Geometry check sheet. Reference: drawing and pictorial views, mm from the part's lowest x, y, z. A direction names the side the tool comes from. Give positions to 0.01 mm unless a question says otherwise; leave off trailing zeros. Loops run counter-clockwise (first coordinate to the right, second up) from the corner with the lowest first, then second, coordinate; pieces in that order, holes last. Notation, with made-up numbers: (-30, 1.5) - (-3, 1.5) arc R15 cw to (-3, 9.5) - close; hole circle Ø6 at (17.25, 16). An arc over 180 degrees is marked (long way). Answer in a Markdown table with one row per item. Add a question column.
(1) Sectioned sample at D-D on x = 28. Enter the section's corners in (y, z).
(2) Set-up check for the marked faces 1 and 2: record each of +Z, -Z, +X, -X, +Y, -Y from which the full face is reachable in a straight line by a thin tool's end or side.
(3) Draft check along Z on the marked faces 3, 4 and 5. Enter one of: released by +Z, released by -Z, zero draft, split by the parting line, or undercut.
(4) Sectioned sample at B-B on x = 16. Enter the section's corners in (y, z).
(5) Sectioned sample at C-C on y = 45. Enter the section's corners in (x, z), then the cut area to 3 significant figures.
(6) Go/stop test with flat-tipped pins: P1, Ø10, axis at y = 44, z = 9.5, coming from the +X side; P2, Ø2, axis at x = 5, y = 51.5, coming from the +Z side; P3, Ø5, axis at x = 18, z = 17, coming from the -Y side; P4, Ø6, axis at y = 9.5, z = 6.5, coming from the -X side. Record where each tip stops, or that it passes through.
(7) Thickness scan on L1, parallel to X at y = 3, z = 16; L2, parallel to Y at x = 18, z = 17.5; L3, parallel to Z at x = 13.5, y = 48. Record the ranges inside material, lowest first.
(8) Sectioned sample at A-A on z = 16. Enter the section's corners in (x, y).
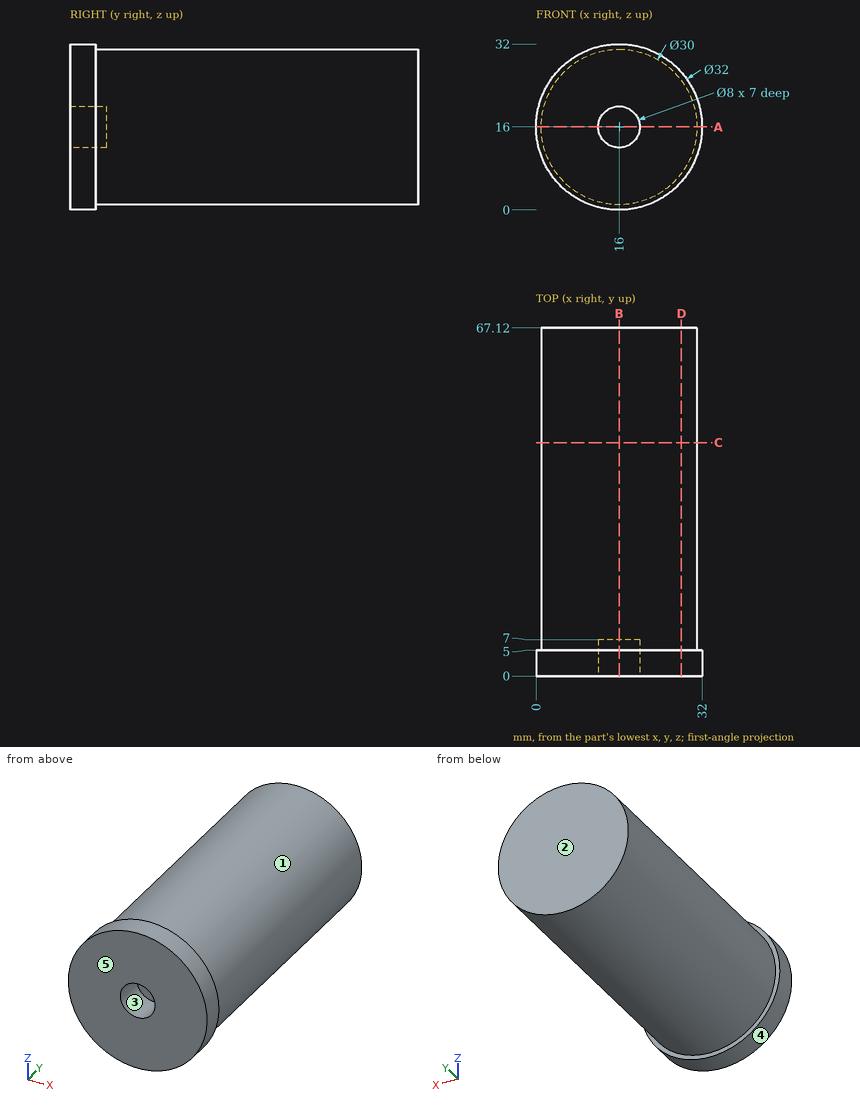
Reply:
| question | item | result |
|---|---|---|
| 1 | outline | (0, 5.42) - (5, 5.42) - (5, 7) - (67.12, 7) - (67.12, 25) - (5, 25) - (5, 26.58) - (0, 26.58) - close |
| 2 | face 1 | +Y |
| 2 | face 2 | +Z, -Z, +X, -X, +Y |
| 3 | face 3 | undercut |
| 3 | face 4 | split by the parting line |
| 3 | face 5 | zero draft |
| 4 | outline | (0, 0) - (5, 0) - (5, 1) - (67.12, 1) - (67.12, 31) - (5, 31) - (5, 32) - (0, 32) - (0, 20) - (7, 20) - (7, 12) - (0, 12) - close |
| 5 | outline | circle Ø30 at (16, 16) |
| 5 | area | 707 mm^2 |
| 6 | P1 | x = 30.92 |
| 6 | P2 | z = 27.18 |
| 6 | P3 | y = 0 |
| 6 | P4 | x = 2.48 |
| 7 | L1 | 0 to 12, 20 to 32 |
| 7 | L2 | 7 to 67.12 |
| 7 | L3 | 1.21 to 30.79 |
| 8 | outline | (0, 0) - (12, 0) - (12, 7) - (20, 7) - (20, 0) - (32, 0) - (32, 5) - (31, 5) - (31, 67.12) - (1, 67.12) - (1, 5) - (0, 5) - close |
